from build123d import *

# Parameters (mm, degrees)
SKETCH_W     = 100
SKETCH_H     = 10
PAD_DEPTH    = 3
SKETCH001_W  = 100
SKETCH001_H  = 3
PAD001_DEPTH = 5
SKETCH002_W  = 100
SKETCH002_H  = 6
PAD002_DEPTH = 3
SKETCH003_W  = 1
SKETCH003_H  = 3
PAD003_DEPTH = 5


with BuildPart() as part:
    # Sketch → Pad (new body)
    with BuildSketch(Plane.XY):
        with Locations((50, 5)):
            Rectangle(SKETCH_W, SKETCH_H)
    extrude(amount=PAD_DEPTH)

    # Sketch001 (on Face6 of Pad) → Pad001 (join)
    with BuildSketch(Plane.XY.offset(3)):
        with Locations((50, 1.5)):
            Rectangle(SKETCH001_W, SKETCH001_H)
    extrude(amount=PAD001_DEPTH)

    # Sketch002 (on Face10 of Pad001) → Pad002 (join)
    with BuildSketch(Plane.XY.offset(8)):
        with Locations((50, 3)):
            Rectangle(SKETCH002_W, SKETCH002_H)
    extrude(amount=PAD002_DEPTH)

    # Sketch003 (on Face15 of Pad002) → Pad003 (join)
    with BuildSketch(Plane(origin=(0, 0, 8), x_dir=(1, 0, 0), z_dir=(0, 0, -1))):
        with Locations((0.5, -4.5)):
            Rectangle(SKETCH003_W, SKETCH003_H)
    extrude(amount=PAD003_DEPTH)


solid = part.part
Here's how the part is built. I have some questions about the finished solid (model axes, mm). A direction names the side the tool comes from. Give positions to 0.01 mm unless a question says otherwise; leave off trailing zeros. Write each loop counter-clockwise with the first axis right and the second up, starting at its lowest first coordinate (ties: lowest second). Pieces come first, ordered by that corner, then holes. Notation, with made-up numbers: (47.5, -30) -> (102.5, -30) arc R24 cw to (102.5, 6) -> close; hole circle Ø3 at (39, 49.5). An arc over 180 degrees is marked (long way). Use one line per item in the form item = value. Start each with the question number.
1. Will these pins go through, and if not, where does the flat tip stop? pin 1 Ø0.9 at (y, z) = (5, 5) entering from +X; pin 2 Ø3 at (y, z) = (8, 5) entering from +X; pin 3 Ø2.5 at (x, z) = (40.5, 6) entering from +Y.
2. Imagine slicing it at C-C on y = 8.75. List the corners of the cut face in (x, z) for me, plus the area to 3 significant figures.
3. Imagine slicing it at A-A on y = 4. List the corners of the cut face in (x, z) for me.
4. Imagine slicing it at B-B on x = 77. List the corners of the cut face in (y, z) for me.
5. On a 3-axis mill with a long thin cutter (end or side, diameter ignored), from which of +Z, -Z, +X, -X, +Y, -Y can I reach the whole of each face in a straight line? I mean faces 5 (the face through (50, 3, 5)), 6 (the face through (50, 6, 10)), 7 (the face through (49, 3, 11)). Say none if no direction works.
6. If I drill on L1, parallel to Z at x = 17.5, y = 4; L2, parallel to Y at x = 77, z = 5.75, over which ranges is the centre line in solid material (lowest first)?
7. Thinking about a two-plate mould opening in Z: for faces 1 (the face through (49, 5, 0)), 2 (the face through (49, 7, 3)), 3 (the face through (50, 5, 8)), 4 (the face through (0, 4, 4)), which applies, +Z half, -Z half, draft (parallel to the pull), parting line (faces both ways), or undercut?
Entries:
q1.pin_1 = 1
q1.pin_2 = through
q1.pin_3 = 3
q2.outline = (0, 0) -> (100, 0) -> (100, 3) -> (0, 3) -> close
q2.area = 300 mm²
q3.outline = (0, 0) -> (100, 0) -> (100, 3) -> (1, 3) -> (1, 8) -> (100, 8) -> (100, 11) -> (0, 11) -> close
q4.outline = (0, 0) -> (10, 0) -> (10, 3) -> (3, 3) -> (3, 8) -> (6, 8) -> (6, 11) -> (0, 11) -> close
q5.face_5 = +X, +Y
q5.face_6 = +Z, +X, -X, +Y
q5.face_7 = +Z, +X, -X, +Y, -Y
q6.L1 = 0 to 3, 8 to 11
q6.L2 = 0 to 3
q7.face_1 = -Z half
q7.face_2 = undercut
q7.face_3 = undercut
q7.face_4 = draft
